Build history of the part. All positions in model axes, mm. Face numbers are marked on the shaded views. A direction names the side the tool comes from. Give positions to 0.01 mm unless a question says otherwise; leave off trailing zeros. Write each loop counter-clockwise with the first axis right and the second up, starting at its lowest first coordinate (ties: lowest second). Pieces come first, ordered by that corner, then holes. Notation, with made-up numbers: (8, 82.25) -> (61, 82.25) arc R9 cw to (61, 96.25) -> close; hole circle Ø9 at (54.5, 45). An arc over 180 degrees is marked (long way). Write item = value, one per line. Start each with the question number.
Q1. Saw through at C-C, the plane y = 29.5. List the corners of the cut face in (x, z).
Q2. Mould opens along Z. For the marked faces 5, 6 and 7 say: pulls with the +Z half, pulls with the -Z half, needs draft (parallel to the pull), parting line crosses it, or undercut.
Q3. Wall check: line 1 (Z direction, x = -15, y = 13.5); line 2 (X direction, y = 1, z = -8); line 3 (Z direction, x = 19, y = 17). Give the ranges that are in metal, low to high.
Q4. Drop flat-ended pins along their axis: P1, Ø13.5, axis at x = 1.5, z = 2.5, coming from the +Y side; P2, Ø12, axis at y = 27, z = -10.5, coming from the -X side; P3, Ø8, axis at x = 3, y = 17, coming from the +Z side; P4, Ø6, axis at x = -14.5, z = 21, coming from the -Y side. Give the stop position or say it passes through.
Q5. Tool access for the marked faces 1, 2, 3 and 4: list every direction of +Z, -Z, +X, -X, +Y, -Y with a clear straight run to the whole face (end or side of a thin tool).
Q6. Saw through at B-B, the plane x = 13.5. List the corners of the cut face in (y, z), then the cut area to 3 significant figures.
Q7. Saw through at D-D, the plane y = 10.5. List the corners of the cut face in (x, z), then the cut area to 3 significant figures.
Q8. Saw through at A-A, the plane z = 12.5. List the corners of the cut face in (x, y).
from build123d import *

# Parameters (mm, degrees)
SKETCH1_W           = 45
SKETCH1_H           = 60
BOSS_EXTRUDE1_DEPTH = 4
SKETCH2_W           = 10
SKETCH2_H           = 3.8
BOSS_EXTRUDE2_DEPTH = 20
CUT_EXTRUDE1_REACH  = 70.427
SKETCH3_R           = 1
CUT_EXTRUDE2_REACH  = 70.427
SKETCH4_R           = 1
SKETCH5_W           = 18
SKETCH5_H           = 15
BOSS_EXTRUDE3_DEPTH = 35
SKETCH6_W           = 13
SKETCH6_H           = 20
CUT_EXTRUDE3_DEPTH  = 6
CUT_EXTRUDE4_REACH  = 77.015
SKETCH7_R           = 1.5
FILLET1_R           = 2
CHAMFER2_SIZE       = 1
CHAMFER3_SIZE       = 1
CUT_EXTRUDE5_REACH  = 56.104
SKETCH8_R           = 1.5
SKETCH8_W           = 12
SKETCH8_H           = 24


with BuildPart() as part:
    # Sketch1 → Boss-Extrude1 (new body)
    with BuildSketch(Plane(origin=(0, 0, 0), x_dir=(1, 0, 0), z_dir=(0, 1, 0))):
        Rectangle(SKETCH1_W, SKETCH1_H)
    extrude(amount=BOSS_EXTRUDE1_DEPTH)

    # Sketch2 → Boss-Extrude2 (add)
    with BuildSketch(Plane(origin=(0, 4, 0), x_dir=(1, 0, 0), z_dir=(0, 1, 0))):
        with Locations((-17.5, 28.1)):
            Rectangle(SKETCH2_W, SKETCH2_H)
        with Locations((-17.5, -28.1)):
            Rectangle(SKETCH2_W, SKETCH2_H)
    extrude(amount=BOSS_EXTRUDE2_DEPTH)

    # Sketch3 → Cut-Extrude1 (cut, up to next)
    with BuildSketch(Plane.XY.offset(30), mode=Mode.PRIVATE) as cut_extrude1_sk1:
        with Locations((-17.5, 19)):
            Circle(SKETCH3_R)
    cut_extrude1_tool1 = extrude(cut_extrude1_sk1.sketch, amount=-CUT_EXTRUDE1_REACH, mode=Mode.PRIVATE) & part.part
    add(cut_extrude1_tool1.solids().sort_by_distance((-17.5, 19, 30))[0], mode=Mode.SUBTRACT)

    # Sketch4 → Cut-Extrude2 (cut, up to next)
    with BuildSketch(Plane(origin=(0, 0, -30), x_dir=(-1, 0, 0), z_dir=(0, 0, -1)), mode=Mode.PRIVATE) as cut_extrude2_sk1:
        with Locations(Location((17.5, 19, 0), (0, 0, 180))):
            Circle(SKETCH4_R)
    cut_extrude2_tool1 = extrude(cut_extrude2_sk1.sketch, amount=-CUT_EXTRUDE2_REACH, mode=Mode.PRIVATE) & part.part
    add(cut_extrude2_tool1.solids().sort_by_distance((-17.5, 19, -30))[0], mode=Mode.SUBTRACT)

    # Sketch5 → Boss-Extrude3 (add)
    with BuildSketch(Plane(origin=(0, 4, 0), x_dir=(1, 0, 0), z_dir=(0, 1, 0))):
        with Locations((13.5, 22.5)):
            Rectangle(SKETCH5_W, SKETCH5_H)
    extrude(amount=BOSS_EXTRUDE3_DEPTH)

    # Sketch6 → Cut-Extrude3 (cut)
    with BuildSketch(Plane(origin=(0, 39, 0), x_dir=(1, 0, 0), z_dir=(0, 1, 0))):
        with Locations((13.5, 20)):
            Rectangle(SKETCH6_W, SKETCH6_H)
    extrude(amount=-CUT_EXTRUDE3_DEPTH, mode=Mode.SUBTRACT)

    # Sketch7 → Cut-Extrude4 (cut, up to next)
    with BuildSketch(Plane(origin=(0, 0, -30), x_dir=(-1, 0, 0), z_dir=(0, 0, -1)), mode=Mode.PRIVATE) as cut_extrude4_sk1:
        with Locations((-13.5, 29.5)):
            Circle(SKETCH7_R)
    cut_extrude4_tool1 = extrude(cut_extrude4_sk1.sketch, amount=-CUT_EXTRUDE4_REACH, mode=Mode.PRIVATE) & part.part
    add(cut_extrude4_tool1.solids().sort_by_distance((13.5, 29.5, -30))[0], mode=Mode.SUBTRACT)

    # Fillet1
    fillet1_edges = [part.edges().sort_by_distance(p)[0] for p in [
        (-12.5, 24, -28.1),
        (-22.5, 24, -28.1),
        (-12.5, 24, 28.1),
        (-22.5, 24, 28.1),
    ]]
    fillet(fillet1_edges, radius=FILLET1_R)

    # Chamfer2
    chamfer2_edges = [part.edges().sort_by_distance(p)[0] for p in [
        (-18.5, 19, -30),
    ]]
    chamfer(chamfer2_edges, length=CHAMFER2_SIZE)

    # Chamfer3
    chamfer3_edges = [part.edges().sort_by_distance(p)[0] for p in [
        (-18.5, 19, 30),
    ]]
    chamfer(chamfer3_edges, length=CHAMFER3_SIZE)

    # Sketch8 → Cut-Extrude5 (cut, up to next)
    with BuildSketch(Plane.XZ, mode=Mode.PRIVATE) as cut_extrude5_sk1:
        with Locations(Location((0, -8, 0), (0, 0, 270))):
            Circle(SKETCH8_R)
    cut_extrude5_tool1 = extrude(cut_extrude5_sk1.sketch, amount=-CUT_EXTRUDE5_REACH, mode=Mode.PRIVATE) & part.part
    # Sketch8 → Cut-Extrude5 (cut, up to next)
    with BuildSketch(Plane.XZ, mode=Mode.PRIVATE) as cut_extrude5_sk2:
        with Locations(Location((0, 20, 0), (0, 0, 270))):
            Circle(SKETCH8_R)
    cut_extrude5_tool2 = extrude(cut_extrude5_sk2.sketch, amount=-CUT_EXTRUDE5_REACH, mode=Mode.PRIVATE) & part.part
    # Sketch8 → Cut-Extrude5 (cut, up to next)
    with BuildSketch(Plane.XZ, mode=Mode.PRIVATE) as cut_extrude5_sk3:
        with Locations((0, 5.960185671)):
            Rectangle(SKETCH8_W, SKETCH8_H)
    cut_extrude5_tool3 = extrude(cut_extrude5_sk3.sketch, amount=-CUT_EXTRUDE5_REACH, mode=Mode.PRIVATE) & part.part
    add(cut_extrude5_tool1.solids().sort_by_distance((0, 0, -8))[0], mode=Mode.SUBTRACT)
    add(cut_extrude5_tool2.solids().sort_by_distance((0, 0, 20))[0], mode=Mode.SUBTRACT)
    add(cut_extrude5_tool3.solids().sort_by_distance((0, 0, 5.960186))[0], mode=Mode.SUBTRACT)


solid = part.part
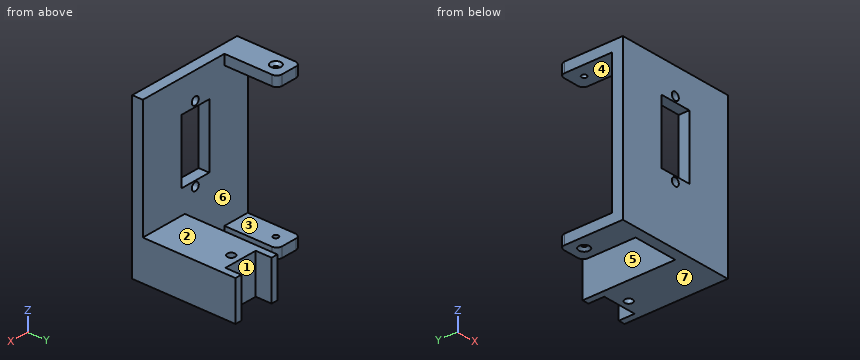
Report:
q1.outline = (4.5, -30) -> (12, -30) -> (12, -15) -> (4.5, -15) -> close; (15, -30) -> (22.5, -30) -> (22.5, -15) -> (15, -15) -> close
q2.face_5 = needs draft
q2.face_6 = undercut
q2.face_7 = pulls with the -Z half
q3.line_1 = -30 to -26.2, 26.2 to 30
q3.line_2 = -22.5 to -1.5, 1.5 to 22.5
q3.line_3 = -30 to -15
q4.P1 = 4
q4.P2 = 4.5
q4.P3 = -15
q4.P4 = 0
q5.face_1 = +Z, -Z, +Y
q5.face_2 = +Z, +X, -X, +Y
q5.face_3 = -X, +Y
q5.face_4 = +X, -X, +Y
q6.outline = (0, -30) -> (28, -30) -> (28, -15) -> (4, -15) -> (4, 30) -> (0, 30) -> close; (31, -30) -> (33, -30) -> (33, -15) -> (31, -15) -> close
q6.area = 630 mm2
q7.outline = (-22.5, -30) -> (-12.5, -30) -> (-12.5, -26.2) -> (-22.5, -26.2) -> close; (-22.5, 26.2) -> (-12.5, 26.2) -> (-12.5, 30) -> (-22.5, 30) -> close; (4.5, -30) -> (22.5, -30) -> (22.5, -15) -> (4.5, -15) -> close
q7.area = 346 mm2
q8.outline = (-22.5, 0) -> (-6, 0) -> (-6, 4) -> (-22.5, 4) -> close; (6, 0) -> (22.5, 0) -> (22.5, 4) -> (6, 4) -> close
